from build123d import *

# Parameters (mm, degrees)
ESBO_O1_W                = 80
ESBO_O1_H                = 80
RESSALTO_EXTRUS_O1_DEPTH = 190
FILETE2_R                = 20
ESBO_O2_R                = 20
RESSALTO_EXTRUS_O2_DEPTH = 25
ESBO_O3_W                = 70
ESBO_O3_H                = 70
CORTE_EXTRUS_O1_DEPTH    = 135
ESBO_O4_R                = 15
CORTE_EXTRUS_O2_DEPTH    = 5


with BuildPart() as part:
    # Esboço1 → Ressalto-extrusão1 (new body)
    with BuildSketch(Plane(origin=(0, 0, 0), x_dir=(1, 0, 0), z_dir=(0, 1, 0))):
        Rectangle(ESBO_O1_W, ESBO_O1_H)
    extrude(amount=RESSALTO_EXTRUS_O1_DEPTH)

    # Filete2
    filete2_edges = [part.edges().sort_by_distance(p)[0] for p in [
        (40, 190, 0),
        (-40, 190, 0),
    ]]
    fillet(filete2_edges, radius=FILETE2_R)

    # Esboço2 → Ressalto-extrusão2 (add)
    with BuildSketch(Plane.XY.offset(40)):
        with Locations(Location((0, 160, 0), (0, 0, 180))):
            Circle(ESBO_O2_R)
    extrude(amount=RESSALTO_EXTRUS_O2_DEPTH)

    # Esboço3 → Corte-extrusão1 (cut)
    with BuildSketch(Plane(origin=(0, 0, 0), x_dir=(-1, 0, 0), z_dir=(0, -1, 0))):
        Rectangle(ESBO_O3_W, ESBO_O3_H)
    extrude(amount=-CORTE_EXTRUS_O1_DEPTH, mode=Mode.SUBTRACT)

    # Esboço4 → Corte-extrusão2 (cut)
    with BuildSketch(Plane.XY.offset(40)):
        with Locations((0, 90)):
            Circle(ESBO_O4_R)
    extrude(amount=-CORTE_EXTRUS_O2_DEPTH, mode=Mode.SUBTRACT)

    # Corte de superfície1
    split(bisect_by=Plane(origin=(0, 135, 0), x_dir=(1, 0, 0), z_dir=(0, 1, 0)), keep=Keep.TOP)


solid = part.part
Model file for the job. Use its own axes, mm. A direction names the side the tool comes from. Give positions to 0.01 mm unless a question says otherwise; leave off trailing zeros. Loops run counter-clockwise (first coordinate to the right, second up) from the corner with the lowest first, then second, coordinate; pieces in that order, holes last.
1) Tool access for faces 1 (the flat face through (-0.6, 180.4, 40)), 2 (the flat face through (-40, 152, 1)): list every direction of +Z, -Z, +X, -X, +Y, -Y with a clear straight run to the whole face (end or side of a thin tool).
2) Saw through at A-A (x = 0). Write the cut outline in (y, z).
3) Flat gauge pin, fed straight in: pin 1 Ø8 at (x, z) = (30, -5.5) entering from +Y. Where does the tip first touch, or does it go through?
4) Saw through at B-B (y = 160). Write the cut outline in (x, z).
5) Saw through at C-C (z = -5). Write the cut outline in (x, y), plus the area to 3 significant figures.
6) Wall check: line 1 (Z direction, x = -6, y = 184); line 2 (Y direction, x = 21, z = 7.5); line 3 (X direction, y = 173.5, z = -21.5). Give the ranges that are in metal, low to high.
Answer block:
1. face 1: +Z
1. face 2: +Z, -Z, -X, +Y, -Y
2. outline: (135, -40) - (190, -40) - (190, 40) - (180, 40) - (180, 65) - (140, 65) - (140, 40) - (135, 40) - close
3. pin 1: stops at y = 189.08
4. outline: (-40, -40) - (40, -40) - (40, 40) - (20, 40) - (20, 65) - (-20, 65) - (-20, 40) - (-40, 40) - close
5. outline: (-40, 135) - (40, 135) - (40, 170) arc R20 ccw to (20, 190) - (-20, 190) arc R20 ccw to (-40, 170) - close
5. area: 4,230 mm2
6. line 1: z = -40 to 40
6. line 2: y = 135 to 189.97
6. line 3: x = -39.69 to 39.69
